Part print with two shaded views. Sizes in mm from the minimum x, y, z corner. Give positions to 0.01 mm unless a question says otherwise; leave off trailing zeros. Write each loop counter-clockwise with the first axis right and the second up, starting at its lowest first coordinate (ties: lowest second). Pieces come first, ordered by that corner, then holes. Notation, with made-up numbers: (55.25, -28.75) -> (99.25, -28.75) arc R28 cw to (99.25, 4.25) -> close; hole circle Ø3 at (10.5, -32.5). An arc over 180 degrees is marked (long way). Answer as a JSON object with one key per item and string values.
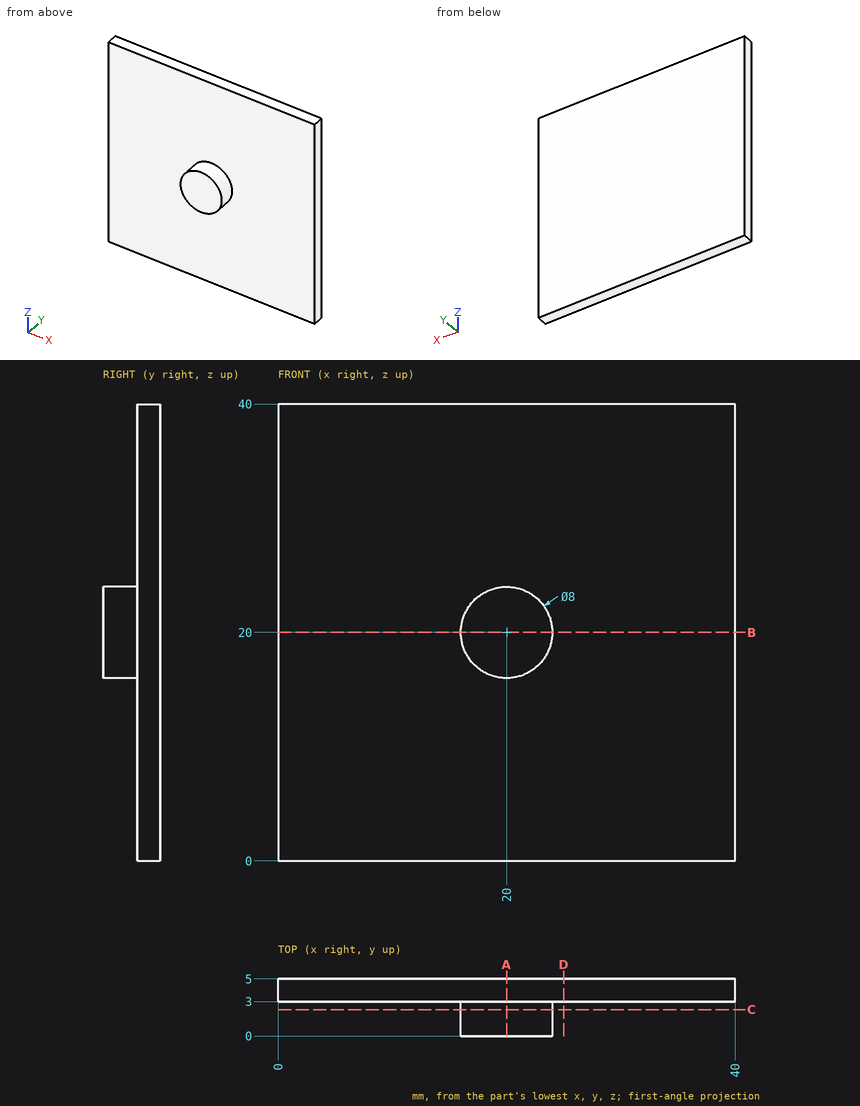
1) Slice it at A-A (x = 20). List the corners of the cut face in (y, z), then the cut area to 3 significant figures.
Model answer:
{"outline": "(0, 16) -> (3, 16) -> (3, 0) -> (5, 0) -> (5, 40) -> (3, 40) -> (3, 24) -> (0, 24) -> close", "area": "104 mm2"}
2) Slice it at C-C (y = 2.3). List the corners of the cut face in (x, z), then the cut area to 3 significant figures.
Model answer:
{"outline": "circle Ø8 at (20, 20)", "area": "50.3 mm2"}
3) Slice it at B-B (z = 20). List the corners of the cut face in (x, y).
Model answer:
{"outline": "(0, 3) -> (16, 3) -> (16, 0) -> (24, 0) -> (24, 3) -> (40, 3) -> (40, 5) -> (0, 5) -> close"}
4) Slice it at D-D (x = 25). List the corners of the cut face in (y, z).
Model answer:
{"outline": "(3, 0) -> (5, 0) -> (5, 40) -> (3, 40) -> close"}
5) Wall check: probe 1 along Y at (x, z) = (11, 27.5); probe 2 along Z at (x, y) = (20, 2.35); probe 3 along X at (y, z) = (1.95, 17). Give the ranges that are in metal, low to high.
Model answer:
{"probe 1": "y = 3 to 5", "probe 2": "z = 16 to 24", "probe 3": "x = 17.35 to 22.65"}
6) Pin check, flat tips, straight feed: pin 1 (1.5 mm diameter, centred on x = 16, y = 1.5, fed in from -Z); pin 2 (12 mm diameter, centred on x = 18.5, z = 36, fed in from -Y). Stop position of each tip, or through.
Model answer:
{"pin 1": "stops at z = 17.67", "pin 2": "stops at y = 3"}
